```python
from build123d import *

# Parameters (mm, degrees)
BOSS_EXTRUDE1_DEPTH = 20
BOSS_EXTRUDE2_DEPTH = 3
SKETCH4_W           = 3
SKETCH4_H           = 7.25
BOSS_EXTRUDE3_DEPTH = 5
SKETCH5_W           = 3.625
SKETCH5_H           = 3
BOSS_EXTRUDE4_DEPTH = 5
SKETCH6_W           = 6
SKETCH6_H           = 84
BOSS_EXTRUDE5_DEPTH = 4


with BuildPart() as part:
    # Sketch2 → Boss-Extrude1 (new body)
    with BuildSketch(Plane.XY):
        Polygon((-17.6, 0), (-17.6, -1.1), (-14.5, -1.1), (-14.5, -5), (-22.5, -5), (-22.5, 0), (-22.5, 4), (22.5, 4), (22.5, -5), (14.5, -5), (14.5, -1.1), (17.6, -1.1), (17.6, 0), align=None)
    extrude(amount=BOSS_EXTRUDE1_DEPTH)

    # Sketch3 → Boss-Extrude2 (add)
    with BuildSketch(Plane(origin=(0, 4, 0), x_dir=(1, 0, 0), z_dir=(0, 1, 0))):
        Polygon((-21.25, -52), (21.25, -52), (21.25, -54), (21.25, -57), (28.5, -57), (28.5, -54), (31.5, -54), (31.5, -46.75), (28.5, -46.75), (28.5, 26.75), (31.5, 26.75), (31.5, 34), (28.5, 34), (28.5, 37), (21.25, 37), (21.25, 34), (21.25, 32), (-21.25, 32), (-21.25, 34), (-21.25, 37), (-28.5, 37), (-28.5, 34), (-31.5, 34), (-31.5, 26.75), (-28.5, 26.75), (-28.5, -46.75), (-31.5, -46.75), (-31.5, -54), (-28.5, -54), (-28.5, -57), (-21.25, -57), (-21.25, -54), align=None)
    extrude(amount=BOSS_EXTRUDE2_DEPTH)

    # Sketch4 → Boss-Extrude3 (add)
    with BuildSketch(Plane(origin=(0, 7, 0), x_dir=(1, 0, 0), z_dir=(0, 1, 0))):
        with Locations((-30, 30.375)):
            Rectangle(SKETCH4_W, SKETCH4_H)
        with Locations((30, 30.375)):
            Rectangle(SKETCH4_W, SKETCH4_H)
        with Locations((30, -50.375)):
            Rectangle(SKETCH4_W, SKETCH4_H)
        with Locations((-30, -50.375)):
            Rectangle(SKETCH4_W, SKETCH4_H)
    extrude(amount=BOSS_EXTRUDE3_DEPTH)

    # Sketch5 → Boss-Extrude4 (add)
    with BuildSketch(Plane(origin=(0, 7, 0), x_dir=(1, 0, 0), z_dir=(0, 1, 0))):
        with Locations((-23.0625, 35.5)):
            Rectangle(SKETCH5_W, SKETCH5_H)
        with Locations((23.0625, 35.5)):
            Rectangle(SKETCH5_W, SKETCH5_H)
        with Locations((23.0625, -55.5)):
            Rectangle(SKETCH5_W, SKETCH5_H)
        with Locations((-23.0625, -55.5)):
            Rectangle(SKETCH5_W, SKETCH5_H)
    extrude(amount=BOSS_EXTRUDE4_DEPTH)

    # Sketch6 → Boss-Extrude5 (add)
    with BuildSketch(Plane.XZ.offset(-4)):
        with Locations((0, 10)):
            Rectangle(SKETCH6_W, SKETCH6_H)
    extrude(amount=BOSS_EXTRUDE5_DEPTH)


solid = part.part
```
Work out the finished part from the listing and answer in its coordinate system (mm). A direction names the side the tool comes from. Give positions to 0.01 mm unless a question says otherwise; leave off trailing zeros. Loops run counter-clockwise (first coordinate to the right, second up) from the corner with the lowest first, then second, coordinate; pieces in that order, holes last. Notation, with made-up numbers: M -2,88.5 L 28,88.5 A6 ccw 28,92.5 Z; hole C -9.5,60.25 d11. An arc over 180 degrees is marked long. One line per item, written item: value. Start each with the question number.
1. Determine the mould class of faces 1 (the face through (-24.875, 9, -35)), 2 (the face through (-28.5, 9, 50)), 3 (the face through (-30, 8, 46.75)) for opening direction X: released by +X, released by -X, zero draft, split by the parting line, or undercut.
2. Find section B-B (z = 7.5). Give the vertices of the cut face in (x, y).
3. Each of these flat-tipped pins is pushed along its axis until it touches: P1, Ø2.5, axis at y = 9, z = -36, coming from the -X side (3 decimals); P2, Ø8, axis at x = 15.5, y = 4, coming from the -Z side; P3, Ø0.9, axis at x = -30.5, y = 7, coming from the -Z side. Where does it stop, or does it pass through?
4. Find section A-A (y = -2.75). Give the vertices of the cut face in (x, z), and give its area (3 significant figures).
5. Find section D-D (y = 5.5). Give the vertices of the cut face in (x, z).
6. Find the intervals of material crossed by probe 1 along X at (y, z) = (7.75, 50); probe 2 along Y at (x, z) = (-0.5, -2.5); probe 3 along Y at (x, z) = (-27.5, 48), in increasing order.
7. Find section C-C (x = 7). Give the vertices of the cut face in (y, z), and give its area (3 significant figures).
8. Which of the six approach directions +Z, -Z, +X, -X, +Y, -Y give full straight-line access (tool end or side, diameter ignored) to faces 4 (the face through (-28.5, 9, -30)), 5 (the face through (-28.5, 5, 9)), 6 (the face through (0, 5, 52)), 7 (the face through (-15, 1, 0)), 8 (the face through (30, 8, -26.75))?
Reported:
1. face 1: released by -X
1. face 2: undercut
1. face 3: zero draft
2. outline: M -28.5,4 L -22.5,4 L -22.5,-5 L -14.5,-5 L -14.5,-1.1 L -17.6,-1.1 L -17.6,0 L 17.6,0 L 17.6,-1.1 L 14.5,-1.1 L 14.5,-5 L 22.5,-5 L 22.5,4 L 28.5,4 L 28.5,7 L -28.5,7 Z
3. P1: stops at x = -24.875
3. P2: stops at z = -32
3. P3: stops at z = -34
4. outline: M -22.5,0 L -14.5,0 L -14.5,20 L -22.5,20 Z; M 14.5,0 L 22.5,0 L 22.5,20 L 14.5,20 Z
4. area: 320 mm²
5. outline: M -31.5,-34 L -28.5,-34 L -28.5,-37 L -21.25,-37 L -21.25,-32 L 21.25,-32 L 21.25,-37 L 28.5,-37 L 28.5,-34 L 31.5,-34 L 31.5,-26.75 L 28.5,-26.75 L 28.5,46.75 L 31.5,46.75 L 31.5,54 L 28.5,54 L 28.5,57 L 21.25,57 L 21.25,52 L -21.25,52 L -21.25,57 L -28.5,57 L -28.5,54 L -31.5,54 L -31.5,46.75 L -28.5,46.75 L -28.5,-26.75 L -31.5,-26.75 Z
6. probe 1: x = -31.5 to -28.5, 28.5 to 31.5
6. probe 2: y = 0 to 7
6. probe 3: y = 4 to 7
7. outline: M 0,0 L 4,0 L 4,-32 L 7,-32 L 7,52 L 4,52 L 4,20 L 0,20 Z
7. area: 332 mm²
8. face 4: +Z, -Z, +Y
8. face 5: -X, +Y, -Y
8. face 6: +Z, +Y, -Y
8. face 7: -Z, -X, -Y
8. face 8: +X, +Y, -Y
